Answer from the drawing. Dimensions are ordinates in mm from the lowest x, y and z of the part. A direction names the side the tool comes from. Give positions to 0.01 mm unless a question says otherwise; leave off trailing zeros. Order: outer loops, then holes, each group sorted by start corner. A loop starts at its lowest first (then second) coordinate and runs counter-clockwise, first axis right, second up.
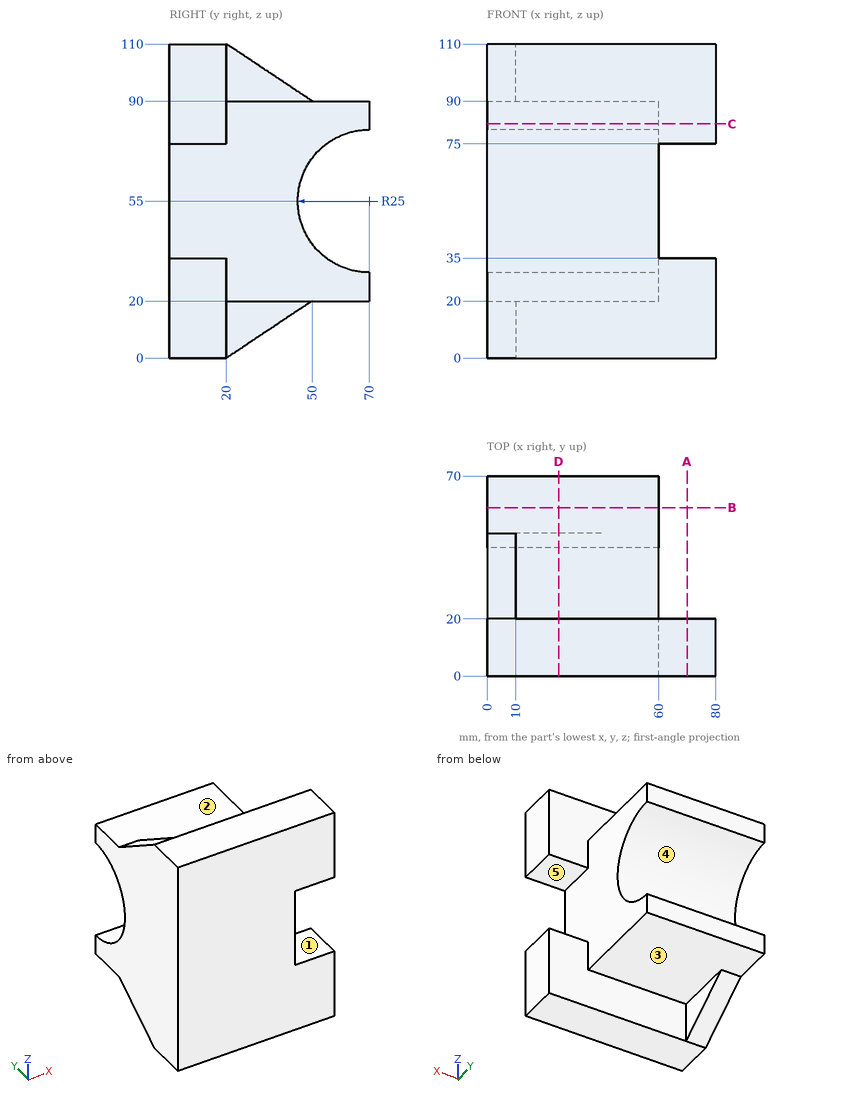
1) Consider L1, parallel to Z at x = 54.5, y = 26; L2, parallel to Y at x = 49, z = 5.5; L3, parallel to X at y = 46, z = 90.5. Determine where each line is inside the solid, lowest interval first.
Final values:
L1: z = 20 to 90
L2: y = 0 to 20
L3: x = 0 to 10
2) For a pull along Z with two mould halves and no side action, classify the marked faces 1, 2 and 3 as released by +Z, released by -Z, zero draft, split by the parting line, or undercut.
Final values:
face 1: undercut
face 2: released by +Z
face 3: released by -Z
3) The part is cut by section B-B on y = 59. Determine the outline of the cut face in (x, z), and give its area (3 significant figures).
Final values:
outline: (0, 20) - (60, 20) - (60, 32.55) - (0, 32.55) - close; (0, 77.45) - (60, 77.45) - (60, 90) - (0, 90) - close
area: 1,510 mm2
4) The part is cut by section C-C on z = 82. Determine the outline of the cut face in (x, y), and give its area (3 significant figures).
Final values:
outline: (0, 0) - (80, 0) - (80, 20) - (60, 20) - (60, 70) - (0, 70) - close
area: 4,600 mm2
5) Given pin 1 (4 mm diameter, centred on x = 62.5, z = 90.5, fed in from +Y); pin 2 (6 mm diameter, centred on y = 31.5, z = 104.5, fed in from +X); pin 3 (1.5 mm diameter, centred on x = 15, z = 70.5, fed in from +Y), each flat-ended and moving along its own axis, determine where each tip first touches the part or whether it passes through.
Final values:
pin 1: stops at y = 20
pin 2: stops at x = 10
pin 3: stops at y = 51
6) The part is cut by section A-A on x = 70. Determine the outline of the cut face in (y, z).
Final values:
outline: (0, 0) - (20, 0) - (20, 35) - (0, 35) - close; (0, 75) - (20, 75) - (20, 110) - (0, 110) - close
7) A tool of negligible diameter and unlimited length cuts with its end or side. For the marked faces 4 and 5, from which of +Z, -Z, +X, -X, +Y, -Y can it reach the whole face along a straight path? Write none if from no direction.
Final values:
face 4: +X, -X, +Y
face 5: +X, +Y, -Y
8) The part is cut by section D-D on x = 25. Determine the outline of the cut face in (y, z), and give its area (3 significant figures).
Final values:
outline: (0, 0) - (20, 0) - (20, 20) - (70, 20) - (70, 30) arc R25 cw to (70, 80) - (70, 90) - (20, 90) - (20, 110) - (0, 110) - close
area: 4,720 mm2
